Part print with two shaded views. Sizes in mm from the minimum x, y, z corner. A direction names the side the tool comes from. Coordinates: 2 decimals unless noted, no trailing zeros. Order: outer loops, then holes, each group sorted by start corner. A loop starts at its lowest first (then second) coordinate and runs counter-clockwise, first axis right, second up. Notation, with made-up numbers: (-28.75, 70.5) - (20.25, 70.5) arc R18 ccw to (20.25, 91.5) - close; hole circle Ø9 at (-22.75, 71.25). An arc over 180 degrees is marked (long way). One line per item, written item: value.
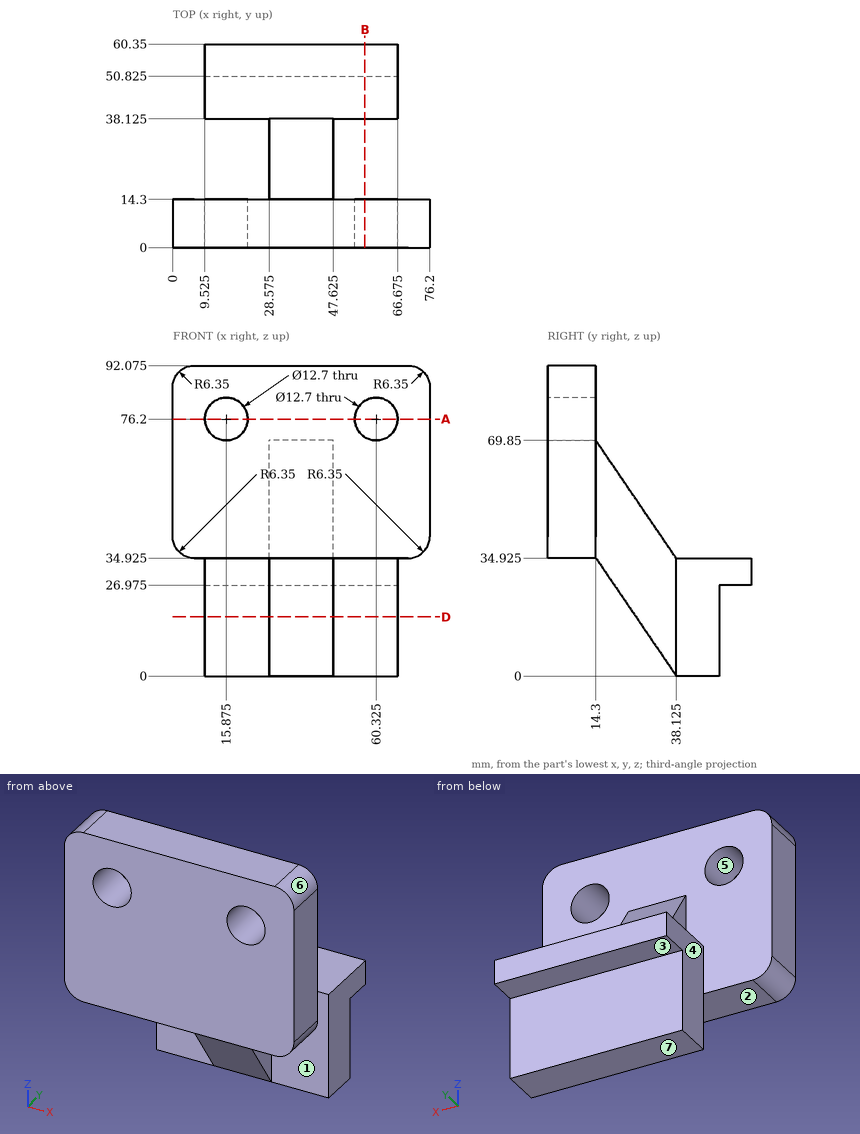
1. Band-saw the part on B-B, the plane x = 57. Count the separate pieces of the cut face and the enclosed holes in it, and give its area (3 significant figures).
Values found:
separate pieces: 3
enclosed holes: 0
area: 1,180 mm2
2. Band-saw the part on A-A, the plane z = 76.2. Give the cut face in (x, y) (1 decimal).
Values found:
outline: (0, 0) - (9.5, 0) - (9.5, 14.3) - (0, 14.3) - close; (22.2, 0) - (54, 0) - (54, 14.3) - (22.2, 14.3) - close; (66.7, 0) - (76.2, 0) - (76.2, 14.3) - (66.7, 14.3) - close
3. Band-saw the part on D-D, the plane z = 17.5. Give the cut face in (x, y) (1 decimal), and give its area (3 significant figures).
Values found:
outline: (9.5, 38.1) - (28.6, 38.1) - (28.6, 26.2) - (47.6, 26.2) - (47.6, 38.1) - (66.7, 38.1) - (66.7, 50.8) - (9.5, 50.8) - close
area: 953 mm2
4. 3-axis set-ups, long thin cutter, end or side, ignore diameter. For the marked faces 1, 2 and 3: which of +Z, -Z, +X, -X, +Y, -Y reach the whole face in a straight line?
Values found:
face 1: +Z, -Z, +X, -Y
face 2: -Z, +X, -X, -Y
face 3: -Z, +X, -X, +Y
5. Two-plate mould, pull along X, no slides. Class the marked faces 4, 5, 6 and 7: pulls with the +X half, pulls with the -X half, needs draft (parallel to the pull), parting line crosses it, or undercut.
Values found:
face 4: pulls with the -X half
face 5: undercut
face 6: pulls with the +X half
face 7: needs draft
6. Flat gauge pins, fed straight in: P1, Ø11, axis at y = 52.5, z = 18.5, coming from the -X side (3 decimals); P2, Ø8, axis at x = 45.5, z = 57, coming from the +Y side (1 decimal); P3, Ø13.5, axis at x = 37, z = 12.5, coming from the +Y side (1 decimal); P4, Ø10, axis at x = 15.875, z = 76.2, coming from the -Y side. Where does each tip first touch, or does it go through?
Values found:
P1: stops at x = 9.525
P2: stops at y = 25.8
P3: stops at y = 50.8
P4: passes through
7. Probe line 1 along X through (y, z) = (3, 76.2) (1 decimal); line 2 along Z through (x, y) = (7, 8) (1 decimal); line 3 along Y through (x, z) = (72.5, 67). List the from-to ranges inside material, lowest first.
Values found:
line 1: x = 0 to 9.5, 22.2 to 54, 66.7 to 76.2
line 2: z = 34.9 to 92.1
line 3: y = 0 to 14.3
